Autodesk Inventor part; units mm, degrees
ref_plane "YZ Plane" through (0, 0, 0) normal (1, 0, 0) x (0, 1, 0)
ref_plane "XZ Plane" through (0, 0, 0) normal (0, 1, 0) x (-1, 0, 0)
ref_plane "XY Plane" through (0, 0, 0) normal (0, 0, 1) x (1, 0, 0)
sketch "Sketch1" plane through (0, 0, 0) normal (0, 1, 0) x (-1, 0, 0)
  circle A0 centre (0, 0) radius 63.5
  circle A1 centre (0, 0) radius 6.35
  circle A2 centre (-12.7, 0) radius 1.75
  circle A3 centre (0, -12.7) radius 1.75
  circle A4 centre (12.7, 0) radius 1.75
  circle A5 centre (0, 12.7) radius 1.75
  dimension "d8" = 3.5
  dimension "d9" = 3.5
  dimension "d10" = 3.5
  dimension "d11" = 3.5
extrude "Extrusion1" add sketch "Sketch1" along normal blind 5.588
sketch "Sketch2" plane through (0, 5.588, 0) normal (0, 1, 0) x (1, 0, 0)
  circle A0 centre (0, 0) radius 63.5
  line L0 (-4.7625, 37.8012) -> (-4.7625, 15.1438)
  line L1 (-4.7625, -15.1438) -> (-4.7625, -37.8012)
  line L2 (4.7625, 37.8012) -> (4.7625, 15.1438)
  line L3 (4.7625, -15.1438) -> (4.7625, -37.8012)
  arc A1 (-4.7625, 37.8012) -> (-4.7625, -37.8012) centre (0, 0) ccw
  arc A2 (4.7625, -37.8012) -> (4.7625, 37.8012) centre (0, 0) ccw
  arc A3 (-4.7625, 15.1438) -> (-4.7625, -15.1438) centre (0, 0) ccw
  arc A4 (4.7625, -15.1438) -> (4.7625, 15.1438) centre (0, 0) ccw
extrude "Extrusion2" cut sketch "Sketch2" against normal blind 25.4 contours L0 A3 L1 A1 | A2 L3 A4 L2
properties part number "AcrylicFlywheel2"
Design review of the part built by this model. Coordinates are the model's own, in mm. A direction names the side the tool comes from. Coordinates: 2 decimals unless noted, no trailing zeros. Order: outer loops, then holes, each group sorted by start corner. A loop starts at its lowest first (then second) coordinate and runs counter-clockwise, first axis right, second up. Notation, with made-up numbers: M 49,67.5 L 105,67.5 A10 cw 105,84.5 Z; hole C 77,55 d8. An arc over 180 degrees is marked long. Use a Markdown table: item, result.
(1) Add section A-A (z = 0). Give the boundary of the cut face in (x, y).
Worked answers:
| item | result |
|---|---|
| outline | M -63.5,0 L -38.1,0 L -38.1,5.59 L -63.5,5.59 Z; M -15.88,0 L -14.45,0 L -14.45,5.59 L -15.88,5.59 Z; M -10.95,0 L -6.35,0 L -6.35,5.59 L -10.95,5.59 Z; M 6.35,0 L 10.95,0 L 10.95,5.59 L 6.35,5.59 Z; M 14.45,0 L 15.88,0 L 15.88,5.59 L 14.45,5.59 Z; M 38.1,0 L 63.5,0 L 63.5,5.59 L 38.1,5.59 Z |
(2) Draft analysis for pull direction X (two halves, no side actions). For faces 1 (the flat face through (1, 5.588, 15)), 2 (the cylindrical face through (-38.092, 2.833, -0.771)), 3 (the cylindrical face through (13.77, 2.75, 61.99)), 4 (the flat face through (4.762, 3, 26)), state which applies: released by +X, released by -X, zero draft, split by the parting line, or undercut.
Worked answers:
| item | result |
|---|---|
| face 1 | zero draft |
| face 2 | undercut |
| face 3 | split by the parting line |
| face 4 | undercut |
(3) Add section C-C (y = 2.55). Give the boundary of the cut face in (x, z).
Worked answers:
| item | result |
|---|---|
| outline | C 0,0 d127; hole C -12.7,0 d3.5; hole C 0,0 d12.7; hole M -4.76,-37.8 L -4.76,-15.14 A15.88 cw -4.76,15.14 L -4.76,37.8 A38.1 ccw Z; hole C 0,-12.7 d3.5; hole C 0,12.7 d3.5; hole M 4.76,-37.8 A38.1 ccw 4.76,37.8 L 4.76,15.14 A15.88 cw 4.76,-15.14 Z; hole C 12.7,0 d3.5 |
(4) For faces 5 (the flat face through (1, 0, 15)), 6 (the flat face through (-4.762, 3, -27)), list the 3-axis set-ups (+Z, -Z, +X, -X, +Y, -Y) from which the entire face can be reached by the end or side of a thin tool; tool diameter is ignored.
Worked answers:
| item | result |
|---|---|
| face 5 | +Z, -Z, +X, -X, -Y |
| face 6 | +Y, -Y |
(5) Wall thickness on probe 1 along Z at (x, y) = (0, 4.35); probe 2 along Z at (x, y) = (-12.7, 4.2); probe 3 along X at (y, z) = (2.5, -9.5): over which ranges is each line inside the solid? List them lowest first.
Worked answers:
| item | result |
|---|---|
| probe 1 | z = -63.5 to -14.45, -10.95 to -6.35, 6.35 to 10.95, 14.45 to 63.5 |
| probe 2 | z = -62.22 to -35.92, -9.53 to -1.75, 1.75 to 9.53, 35.92 to 62.22 |
| probe 3 | x = -62.79 to -36.9, -12.72 to 12.72, 36.9 to 62.79 |
(6) Add section D-D (z = -32.5). Give the boundary of the cut face in (x, y).
Worked answers:
| item | result |
|---|---|
| outline | M -54.55,0 L -19.88,0 L -19.88,5.59 L -54.55,5.59 Z; M -4.76,0 L 4.76,0 L 4.76,5.59 L -4.76,5.59 Z; M 19.88,0 L 54.55,0 L 54.55,5.59 L 19.88,5.59 Z |
(7) Add section B-B (x = 0). Give the boundary of the cut face in (y, z), then the cut area to 3 significant figures.
Worked answers:
| item | result |
|---|---|
| outline | M 0,-63.5 L 5.59,-63.5 L 5.59,-14.45 L 0,-14.45 Z; M 0,-10.95 L 5.59,-10.95 L 5.59,-6.35 L 0,-6.35 Z; M 0,6.35 L 5.59,6.35 L 5.59,10.95 L 0,10.95 Z; M 0,14.45 L 5.59,14.45 L 5.59,63.5 L 0,63.5 Z |
| area | 600 mm2 |
(8) For P1, Ø1.7, axis at y = 4, z = 29, coming from the -X side; P2, Ø1.7, axis at y = 2.5, z = 29, coming from the +X side; P3, Ø1.5, axis at y = 4.5, z = 17.5, coming from the +X side, all flat-tipped, find the tip position at first contact; note any pin that passes through.
Worked answers:
| item | result |
|---|---|
| P1 | stops at x = -56.92 |
| P2 | stops at x = 56.92 |
| P3 | stops at x = 61.25 |
